CAD build for the part. Positions are in the model's coordinates, mm. Coordinates: 2 decimals unless noted, no trailing zeros. Order: outer loops, then holes, each group sorted by start corner. A loop starts at its lowest first (then second) coordinate and runs counter-clockwise, first axis right, second up. Notation, with made-up numbers: M 83.5,17.25 L 93.5,17.25 A31 cw 93.5,48.25 Z; hole C 84.5,74.5 d8. An arc over 180 degrees is marked long. Write item = value, one per line.
from build123d import *

# Parameters (mm, degrees)
F0_R     = 10
F1_DEPTH = 5
F4_R     = 8
F5_DEPTH = 2
F6_R     = 0.99999


# Not quite as in the source:
# - a fillet or chamfer is up to 0.001 mm smaller than in the source, because OpenCascade refuses the exact size


with BuildPart() as f1:
    # F0 (on Top) → F1 (new body)
    with BuildSketch(Plane.XY):
        Circle(F0_R)
    extrude(amount=F1_DEPTH)

    # F2 (on Front) → F3 (revolve, cut)
    with BuildSketch(Plane.XZ):
        Polygon((-8, 5), (0, 2.5), (0, 5), align=None)
    revolve(axis=Axis((0, 0, 3.75), (0, 0, -1)), mode=Mode.SUBTRACT)

    # F4 (on face) → F5 (join)
    with BuildSketch(Plane(origin=(0, 0, 0), x_dir=(1, 0, 0), z_dir=(0, 0, -1))):
        Circle(F4_R)
    extrude(amount=F5_DEPTH)

    # F6 (radius 1 in the source; OpenCascade refuses exactly that, so slightly less here)
    f6_edges = [f1.edges().sort_by_distance(p)[0] for p in [
        (-8, 0, 0),
        (-10, 0, 0),
        (-10, 0, 5),
        (8, 0, 5),
    ]]
    fillet(f6_edges, radius=F6_R)


solid = f1.part
(1) Slice it at B-B, the plane z = -0.5. Write the cut outline in (x, y).
Evaluation:
outline = C 0,0 d16.27
(2) Pull direction X, two halves, no side cores. Call faces 1 (the face through (0.08, -0.37, 2.62)), 2 (the face through (0, 0, -2)), 3 (the face through (-1.73, 7.81, -1.49)): +X half, -X half, draft (parallel to the pull), parting line (faces both ways), or undercut.
Evaluation:
face_1 = undercut
face_2 = draft
face_3 = parting line
(3) Slice it at A-A, the plane z = 2.75. Write the cut outline in (x, y), then the cut area to 3 significant figures.
Evaluation:
outline = C 0,0 d20; hole C 0,0 d1.6
area = 312 mm²
(4) Pin check, flat tips, straight feed: pin 1 Ø1 at (y, z) = (6, 0) entering from -X; pin 2 Ø1.5 at (y, z) = (4, 0.5) entering from -X; pin 3 Ø4 at (y, z) = (-6.5, 0.5) entering from +X. Stop position of each tip, or through.
Evaluation:
pin_1 = -7.97
pin_2 = -9.42
pin_3 = 8.9
(5) Wall check: line 1 (Z direction, x = -7, y = -1.25); line 2 (Z direction, x = -4, y = -4); line 3 (X direction, y = -6.75, z = 3.5). Give the ranges that are in metal, low to high. Write a range as from..to.
Evaluation:
line_1 = -2..4.72
line_2 = -2..4.27
line_3 = -7.38..7.38
